from build123d import *

# Parameters (mm, degrees)
BOSS_EXTRUDE1_DEPTH = 5
CHAMFER1_SIZE       = 2
CHAMFER2_SIZE       = 6
CHAMFER3_SIZE       = 4


with BuildPart() as part:
    # Sketch2 → Boss-Extrude1 (new body)
    with BuildSketch(Plane(origin=(0, 0, 0), x_dir=(1, 0, 0), z_dir=(0, 1, 0))):
        Polygon((40.026305405, 0), (0.026305405, 0), (0.026305405, -8), (40.026305405, -8), (40.026305405, -38), (53.026305405, -38), (53.026305405, -32), (55.026305405, -30), (61.026305405, -30), (61.026305405, -15), align=None)
        with BuildLine():
            ThreePointArc((47.026305405, -27.5), (45.526305405, -26), (47.026305405, -24.5))
            Line((47.026305405, -24.5), (53.026305405, -24.5))
            ThreePointArc((53.026305405, -24.5), (54.526305405, -26), (53.026305405, -27.5))
            Line((53.026305405, -27.5), (47.026305405, -27.5))
        make_face(mode=Mode.SUBTRACT)
        with BuildLine():
            ThreePointArc((47.026305405, -21.5), (45.526305405, -20), (47.026305405, -18.5))
            Line((47.026305405, -18.5), (53.026305405, -18.5))
            ThreePointArc((53.026305405, -18.5), (54.526305405, -20), (53.026305405, -21.5))
            Line((53.026305405, -21.5), (47.026305405, -21.5))
        make_face(mode=Mode.SUBTRACT)
        with BuildLine():
            ThreePointArc((9.026305405, -5.5), (7.526305405, -4), (9.026305405, -2.5))
            Line((9.026305405, -2.5), (15.026305405, -2.5))
            ThreePointArc((15.026305405, -2.5), (16.526305405, -4), (15.026305405, -5.5))
            Line((15.026305405, -5.5), (9.026305405, -5.5))
        make_face(mode=Mode.SUBTRACT)
        with BuildLine():
            ThreePointArc((19.026305405, -5.5), (17.526305405, -4), (19.026305405, -2.5))
            Line((19.026305405, -2.5), (25.026305405, -2.5))
            ThreePointArc((25.026305405, -2.5), (26.526305405, -4), (25.026305405, -5.5))
            Line((25.026305405, -5.5), (19.026305405, -5.5))
        make_face(mode=Mode.SUBTRACT)
        with BuildLine():
            ThreePointArc((43.759423492, -11.240077261), (43.562000753, -9.127963566), (45.674114448, -8.930540827))
            Line((45.674114448, -8.930540827), (50.293187317, -12.759922739))
            ThreePointArc((50.293187317, -12.759922739), (50.490610056, -14.872036434), (48.378496361, -15.069459173))
            Line((48.378496361, -15.069459173), (43.759423492, -11.240077261))
        make_face(mode=Mode.SUBTRACT)
        with BuildLine():
            ThreePointArc((29.026305405, -5.5), (27.526305405, -4), (29.026305405, -2.5))
            Line((29.026305405, -2.5), (35.026305405, -2.5))
            ThreePointArc((35.026305405, -2.5), (36.526305405, -4), (35.026305405, -5.5))
            Line((35.026305405, -5.5), (29.026305405, -5.5))
        make_face(mode=Mode.SUBTRACT)
    extrude(amount=BOSS_EXTRUDE1_DEPTH)

    # Chamfer1
    chamfer1_edges = [part.edges().sort_by_distance(p)[0] for p in [
        (0.026305405, 2.5, 8),
        (0.026305405, 2.5, 0),
    ]]
    chamfer(chamfer1_edges, length=CHAMFER1_SIZE)

    # Chamfer2
    chamfer2_edges = [part.edges().sort_by_distance(p)[0] for p in [
        (40.026305405, 2.5, 38),
    ]]
    chamfer(chamfer2_edges, length=CHAMFER2_SIZE)

    # Chamfer3
    chamfer3_edges = [part.edges().sort_by_distance(p)[0] for p in [
        (40.026305405, 2.5, 8),
    ]]
    chamfer(chamfer3_edges, length=CHAMFER3_SIZE)


solid = part.part
Design review of the part built by this model. Coordinates are the model's own, in mm. A direction names the side the tool comes from. Give positions to 0.01 mm unless a question says otherwise; leave off trailing zeros. Write each loop counter-clockwise with the first axis right and the second up, starting at its lowest first coordinate (ties: lowest second). Pieces come first, ordered by that corner, then holes. Notation, with made-up numbers: M 20.5,-7 L 71.5,-7 A26 cw 71.5,21 Z; hole C 5.5,18.5 d7. An arc over 180 degrees is marked long. Return JSON: item names as keys, results as strings. Group by question number.
Item 1: Take a section at B-B (x = 23). Give the boundary of the cut face in (y, z), plus the area to 3 significant figures.
Item 2: Take a section at A-A (z = 20). Give the boundary of the cut face in (x, y).
Item 3: Take a section at C-C (z = 4). Give the boundary of the cut face in (x, y).
Item 4: Wall thickness on line 1 along X through (y, z) = (4.75, 20); line 2 along Z through (x, y) = (32.5, 1.4); line 3 along Z through (x, y) = (49.5, 3.9): over which ranges is each line inside the solid? List them lowest first.
Item 5: Tool access review of faces 1 (the flat face through (19, 2, 8)), 2 (the flat face through (32, 2, 5.5)), 3 (the flat face through (58, 2, 30)): name each direction out of +Z, -Z, +X, -X, +Y, -Y from which nothing blocks a thin tool from reaching the whole face with its end or side.
Item 6: Take a section at D-D (y = 1.75). Count the separate pieces of the cut face and the enclosed holes in it, plus the area to 3 significant figures.
Item 7: Clearance check with flat-ended pins moving along their axes: pin 1 Ø1.5 at (y, z) = (4, 4.5) entering from +X; pin 2 Ø2.5 at (x, y) = (58, 2) entering from +Z; pin 3 Ø2.5 at (x, y) = (51, 3.5) entering from -Z. State where each tip first meets the part, or that it passes through.
Return value:
{
 "1": {"outline": "M 0,0 L 5,0 L 5,2.5 L 0,2.5 Z; M 0,5.5 L 5,5.5 L 5,8 L 0,8 Z", "area": "25.0 mm2"},
 "2": {"outline": "M 40.03,0 L 45.53,0 L 45.53,5 L 40.03,5 Z; M 54.53,0 L 61.03,0 L 61.03,5 L 54.53,5 Z"},
 "3": {"outline": "M 0.03,0 L 7.53,0 L 7.53,5 L 0.03,5 Z; M 16.53,0 L 17.53,0 L 17.53,5 L 16.53,5 Z; M 26.53,0 L 27.53,0 L 27.53,5 L 26.53,5 Z; M 36.53,0 L 45.63,0 L 45.63,5 L 36.53,5 Z"},
 "4": {"line 1": "x = 40.03 to 45.53, 54.53 to 61.03", "line 2": "z = 0 to 2.5, 5.5 to 8", "line 3": "z = 6.77 to 12.1, 15.41 to 18.5, 21.5 to 24.5, 27.5 to 38"},
 "5": {"face 1": "+Z, -X, +Y, -Y", "face 2": "+Y, -Y", "face 3": "+Z, +X, +Y, -Y"},
 "6": {"separate pieces": "1", "enclosed holes": "6", "area": "734 mm2"},
 "7": {"pin 1": "stops at x = 47.38", "pin 2": "stops at z = 30", "pin 3": "stops at z = 6.95"}
}
